Verification items for this drawing (mm, ordinates from the low corner). A direction names the side the tool comes from. Round coordinates to 2 decimals unless told otherwise and drop trailing zeros. Order: outer loops, then holes, each group sorted by start corner. A loop starts at its lowest first (then second) coordinate and runs counter-clockwise, first axis right, second up.
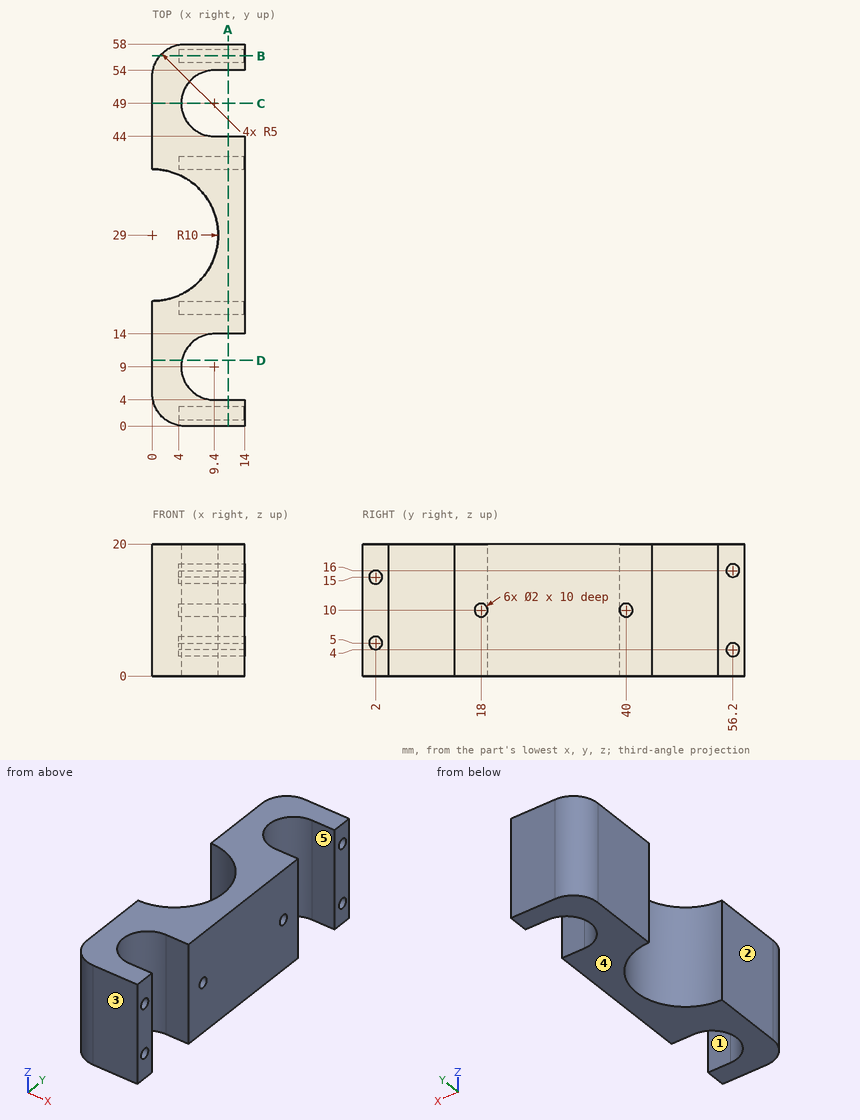
Item 1: Sectioned sample at C-C (y = 49). Record the cut outline in (x, z).
Answer:
outline: (0, 0) - (4.4, 0) - (4.4, 20) - (0, 20) - close
Item 2: Release check for a two-part mould opening along Y. For the marked faces 3, 4 and 5 record: released by +Y, released by -Y, zero draft, split by the parting line, or undercut.
Answer:
face 3: released by -Y
face 4: zero draft
face 5: undercut
Item 3: Scan lines: line 1 along Y through (x, z) = (10.75, 10); line 2 along Y through (x, z) = (12.75, 18.5); line 3 along Z through (x, y) = (6, 40). Record each from-to range of solid material in increasing order.
Answer:
line 1: y = 0 to 4, 14 to 17, 19 to 39, 41 to 44, 54 to 58
line 2: y = 0 to 4, 14 to 44, 54 to 58
line 3: z = 0 to 9, 11 to 20
Item 4: Access from +Z, -Z, +X, -X, +Y, -Y to the whole of each face (thin tool, end or side, straight path). Record for the marked faces 1 and 2.
Answer:
face 1: +Z, -Z, +X
face 2: +Z, -Z, -X, +Y, -Y
Item 5: Sectioned sample at D-D (y = 10). Record the cut outline in (x, z), and give its area (3 significant figures).
Answer:
outline: (0, 0) - (4.5, 0) - (4.5, 20) - (0, 20) - close
area: 90.0 mm2
Item 6: Sectioned sample at B-B (y = 56.2). Record the cut outline in (x, z), and give its area (3 significant figures).
Answer:
outline: (1.16, 0) - (14, 0) - (14, 3) - (4, 3) - (4, 5) - (14, 5) - (14, 15) - (4, 15) - (4, 17) - (14, 17) - (14, 20) - (1.16, 20) - close
area: 217 mm2
Item 7: Sectioned sample at A-A (x = 11.5). State how many separate pieces and enclosed holes the cut face has, and give its area (3 significant figures).
Answer:
separate pieces: 3
enclosed holes: 6
area: 741 mm2
Item 8: Go/stop test with flat-tipped pins: P1, Ø1.8, axis at y = 2, z = 5, coming from the -X side; P2, Ø2.5, axis at y = 56.2, z = 16, coming from the +X side; P3, Ø1.2, axis at y = 40, z = 10, coming from the +X side; P4, Ø2.5, axis at y = 2, z = 15, coming from the -X side. Record where each tip stops, or that it passes through.
Answer:
P1: stops at x = 0.46
P2: stops at x = 14
P3: stops at x = 4
P4: stops at x = 0.32
